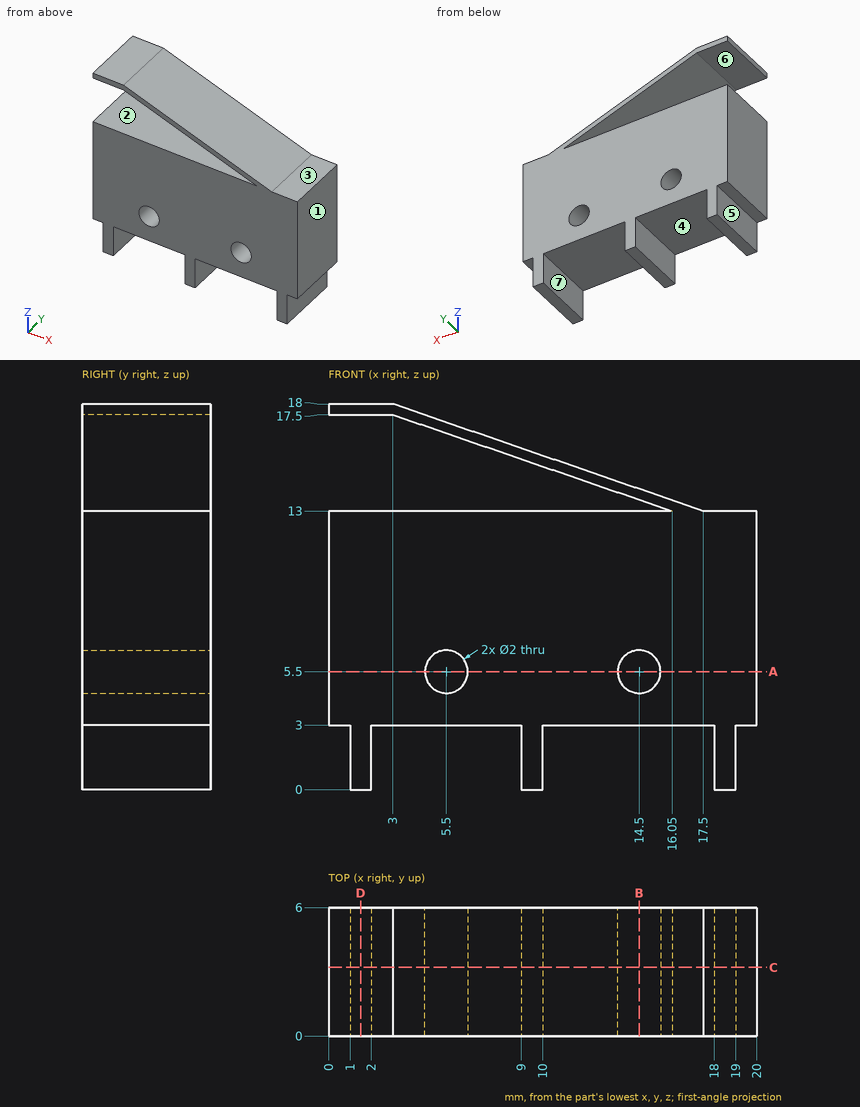
For this review, use the dimensioned drawing (mm, ordinates from the lowest corner) and the shaded views. A direction names the side the tool comes from. Give positions to 0.01 mm unless a question says otherwise; leave off trailing zeros. Write each loop counter-clockwise with the first axis right and the second up, starting at its lowest first coordinate (ties: lowest second). Pieces come first, ordered by that corner, then holes.
(1) Tool access review of the marked faces 5, 6 and 7: name each direction out of +Z, -Z, +X, -X, +Y, -Y from which nothing blocks a thin tool from reaching the whole face with its end or side.
(2) The part is to be moulded in two halves that separate along Z. For the marked faces 1, 2, 3 and 4, say which applies: released by +Z, released by -Z, zero draft, split by the parting line, or undercut.
(3) To check wall thickness, follow L1, parallel to X at y = 2.25, z = 0.5; L2, parallel to Z at x = 5.5, y = 4.4; L3, parallel to Z at x = 14, y = 5.75. State the ranges of each line that lie inside material, in increasing order.
(4) Consider section A-A, the plane z = 5.5. Give the boundary of the cut face in (x, y).
(5) Consider section C-C, the plane y = 3.2. Give the boundary of the cut face in (x, z), and give its area (3 significant figures).
(6) Consider section B-B, the plane x = 14.5. Give the boundary of the cut face in (y, z).
(7) Consider section D-D, the plane x = 1.5. Give the boundary of the cut face in (y, z), and give its area (3 significant figures).
(8) For P1, Ø3, axis at x = 13.5, y = 2.5, coming from the -Z side; P2, Ø0.9, axis at y = 3.5, z = 1, coming from the +X side; P3, Ø1.5, axis at x = 12.5, z = 16, coming from the +Y side; P4, Ø1.5, axis at y = 2.5, z = 2, coming from the -X side, all flat-tipped, find the tip position at first contact; note any pin that passes through.
Returned:
1. face 5: -Z, -X, +Y, -Y
1. face 6: -X, +Y, -Y
1. face 7: -Z, +Y, -Y
2. face 1: zero draft
2. face 2: undercut
2. face 3: released by +Z
2. face 4: released by -Z
3. L1: x = 1 to 2, 9 to 10, 18 to 19
3. L2: z = 3 to 4.5, 6.5 to 13, 16.64 to 17.14
3. L3: z = 3 to 4.63, 6.37 to 13, 13.71 to 14.21
4. outline: (0, 0) - (4.5, 0) - (4.5, 6) - (0, 6) - close; (6.5, 0) - (13.5, 0) - (13.5, 6) - (6.5, 6) - close; (15.5, 0) - (20, 0) - (20, 6) - (15.5, 6) - close
5. outline: (0, 3) - (1, 3) - (1, 0) - (2, 0) - (2, 3) - (9, 3) - (9, 0) - (10, 0) - (10, 3) - (18, 3) - (18, 0) - (19, 0) - (19, 3) - (20, 3) - (20, 13) - (17.5, 13) - (3, 18) - (0, 18) - (0, 17.5) - (3, 17.5) - (16.05, 13) - (0, 13) - close; hole circle Ø2 at (5.5, 5.5); hole circle Ø2 at (14.5, 5.5)
5. area: 211 mm2
6. outline: (0, 3) - (6, 3) - (6, 4.5) - (0, 4.5) - close; (0, 6.5) - (6, 6.5) - (6, 13) - (0, 13) - close; (0, 13.53) - (6, 13.53) - (6, 14.03) - (0, 14.03) - close
7. outline: (0, 0) - (6, 0) - (6, 13) - (0, 13) - close; (0, 17.5) - (6, 17.5) - (6, 18) - (0, 18) - close
7. area: 81.0 mm2
8. P1: stops at z = 3
8. P2: stops at x = 19
8. P3: passes through
8. P4: stops at x = 1
